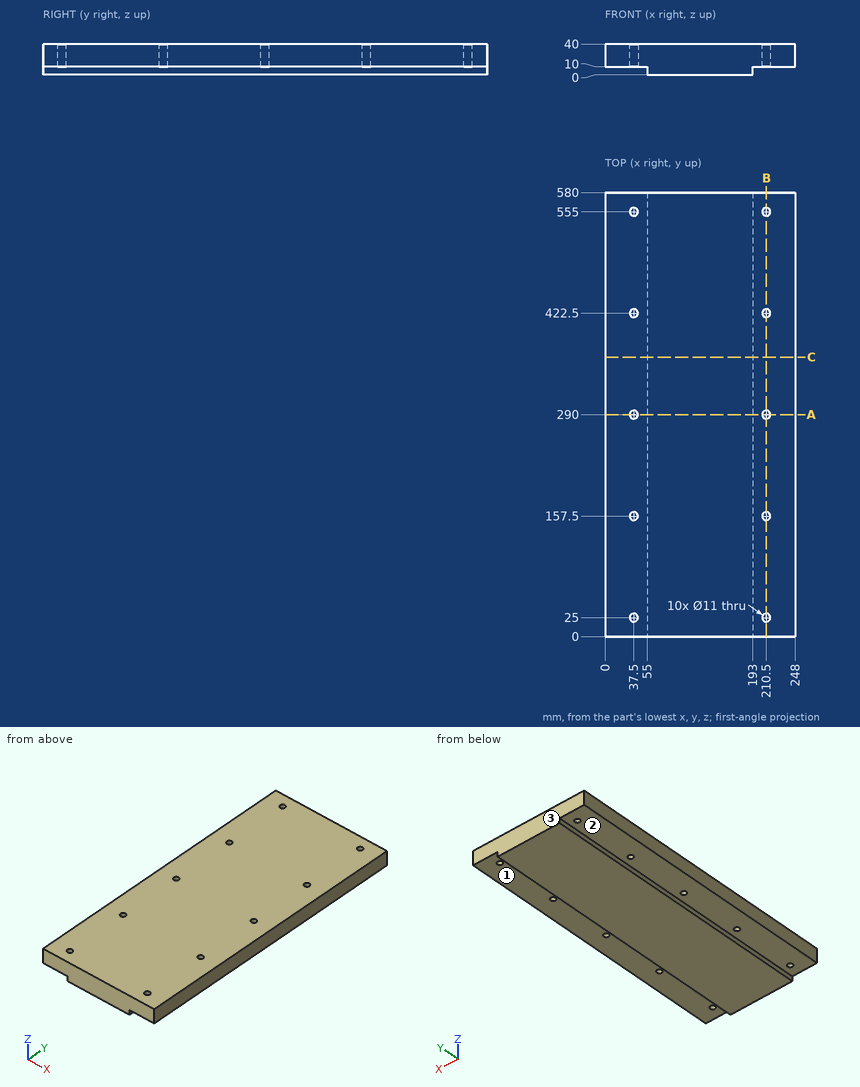
Study the drawing (mm; zero at the part's minimum x, y, z) and answer. A direction names the side the tool comes from. Give positions to 0.01 mm unless a question says otherwise; leave off trailing zeros. Write each loop counter-clockwise with the first axis right and the second up, starting at its lowest first coordinate (ties: lowest second). Pieces come first, ordered by that corner, then holes. Notation, with made-up numbers: M 60.5,6.25 L 67.5,6.25 A25 ccw 67.5,34.25 Z; hole C 86,-27.5 d7. An arc over 180 degrees is marked long. Put each result on its own line as item: value. Start each with the question number.
1. The part is cut by section C-C, the plane y = 365. Give the vertices of the cut face in (x, z).
2. Which of the six approach directions +Z, -Z, +X, -X, +Y, -Y give full straight-line access (tool end or side, diameter ignored) to the marked faces 1, 2 and 3?
3. Each of these flat-tipped pins is pushed along its axis until it touches: pin 1 Ø9 at (x, y) = (210.5, 157.5) entering from -Z; pin 2 Ø14.5 at (x, y) = (37.5, 25) entering from -Z; pin 3 Ø11 at (y, z) = (341, 3.5) entering from -X; pin 4 Ø8 at (y, z) = (351.5, 4.5) entering from +X. Where does it stop, or does it pass through?
4. The part is cut by section A-A, the plane y = 290. Give the vertices of the cut face in (x, z), and give its area (3 significant figures).
5. The part is cut by section B-B, the plane x = 210.5. Give the vertices of the cut face in (y, z).
6. Consider line 1 along Y through (x, z) = (210, 29); line 2 along X through (y, z) = (25, 29); line 3 along X through (y, z) = (159.5, 29.5). Determine where each line is inside the solid, lowest interval first.
Final values:
1. outline: M 0,10 L 55,10 L 55,0 L 193,0 L 193,10 L 248,10 L 248,40 L 0,40 Z
2. face 1: -Z, +X, +Y, -Y
2. face 2: -Z, -X, +Y, -Y
2. face 3: +Z, -Z, +X, -X, +Y
3. pin 1: passes through
3. pin 2: stops at z = 10
3. pin 3: stops at x = 55
3. pin 4: stops at x = 193
4. outline: M 0,10 L 32,10 L 32,40 L 0,40 Z; M 43,10 L 55,10 L 55,0 L 193,0 L 193,10 L 205,10 L 205,40 L 43,40 Z; M 216,10 L 248,10 L 248,40 L 216,40 Z
4. area: 8,160 mm²
5. outline: M 0,10 L 19.5,10 L 19.5,40 L 0,40 Z; M 30.5,10 L 152,10 L 152,40 L 30.5,40 Z; M 163,10 L 284.5,10 L 284.5,40 L 163,40 Z; M 295.5,10 L 417,10 L 417,40 L 295.5,40 Z; M 428,10 L 549.5,10 L 549.5,40 L 428,40 Z; M 560.5,10 L 580,10 L 580,40 L 560.5,40 Z
6. line 1: y = 0 to 19.52, 30.48 to 152.02, 162.98 to 284.52, 295.48 to 417.02, 427.98 to 549.52, 560.48 to 580
6. line 2: x = 0 to 32, 43 to 205, 216 to 248
6. line 3: x = 0 to 32.38, 42.62 to 205.38, 215.62 to 248
